```python
from build123d import *

# Parameters (mm, degrees)
FILLET1_R = 1.5


with BuildPart() as part:
    # Sketch1 → Revolve1 (revolve)
    with BuildSketch(Plane.XY):
        Polygon((33.75, 0), (33.75, -9), (13.25, -9), (13.25, -19), (0, -19), (0, -17), (11.25, -17), (11.25, -7), (31.75, -7), (31.75, 3), (32.75, 3), (32.75, 0), align=None)
    revolve(axis=Axis((0, -19, 0), (0, 1, 0)))

    # Fillet1
    fillet1_edges = [part.edges().sort_by_distance(p)[0] for p in [
        (-13.25, -19, 0),
        (-33.75, -9, 0),
    ]]
    fillet(fillet1_edges, radius=FILLET1_R)


solid = part.part
```
The listing builds one solid part. Answer for the finished solid, in the listing's coordinates (mm). A direction names the side the tool comes from. Coordinates: 2 decimals unless noted, no trailing zeros. Loops run counter-clockwise (first coordinate to the right, second up) from the corner with the lowest first, then second, coordinate; pieces in that order, holes last. Notation, with made-up numbers: (48, 8) -> (92, 8) arc R27 cw to (92, 27) -> close; hole circle Ø4 at (18.5, 13.5). An arc over 180 degrees is marked (long way). Use one line per item in the form item = value. Start each with the question number.
Item 1: A tool of negligible diameter and unlimited length cuts with its end or side. For faces 1 (the face through (0, -19, 0)), 2 (the face through (28, 0, -18)), 3 (the face through (14, -9, 0)), from which of +Z, -Z, +X, -X, +Y, -Y can it reach the whole face along a straight path? Write none if from no direction.
Item 2: The part is cut by section A-A on z = 0. Determine the outline of the cut face in (x, y).
Item 3: The part is cut by section C-C on y = -5.75. Determine the outline of the cut face in (x, z).
Item 4: The part is cut by section D-D on y = -11. Determine the outline of the cut face in (x, z).
Item 5: The mould has two halves that part along Z. Classify faces 4 (the face through (7.123, -13.31, -11.172)), 5 (the face through (0, -17, 0)), 6 (the face through (17, 3, -27)): released by +Z, released by -Z, zero draft, split by the parting line, or undercut.
Item 6: The part is cut by section B-B on x = 0. Determine the outline of the cut face in (y, z), then the cut area to 3 significant figures.
Item 7: Flat-ended cylindrical pins translate along their axes: pin 1 Ø6 at (y, z) = (0.5, 16) entering from -X; pin 2 Ø18 at (x, z) = (0, 0) entering from +Y; pin 3 Ø6 at (x, y) = (14.5, -10) entering from +Z. Find the tip coordinate at first contact, or state that the pin passes through.
Item 8: Consider L1, parallel to X at y = -13.5, z = 0; L2, parallel to Z at x = 0, y = -4. Determine where each line is inside the solid, lowest interval first. Write a range as [from, to].
Answer key:
q1.face_1 = +Z, -Z, +X, -X, -Y
q1.face_2 = +Y
q1.face_3 = -Y
q2.outline = (-33.75, -7.5) arc R1.5 ccw to (-32.25, -9) -> (-13.25, -9) -> (-13.25, -17.5) arc R1.5 ccw to (-11.75, -19) -> (11.75, -19) arc R1.5 ccw to (13.25, -17.5) -> (13.25, -9) -> (32.25, -9) arc R1.5 ccw to (33.75, -7.5) -> (33.75, 0) -> (32.75, 0) -> (32.75, 3) -> (31.75, 3) -> (31.75, -7) -> (11.25, -7) -> (11.25, -17) -> (-11.25, -17) -> (-11.25, -7) -> (-31.75, -7) -> (-31.75, 3) -> (-32.75, 3) -> (-32.75, 0) -> (-33.75, 0) -> close
q3.outline = circle Ø67.5 at (0, 0); hole circle Ø63.5 at (0, 0)
q4.outline = circle Ø26.5 at (0, 0); hole circle Ø22.5 at (0, 0)
q5.face_4 = split by the parting line
q5.face_5 = undercut
q5.face_6 = zero draft
q6.outline = (-19, -11.75) arc R1.5 ccw to (-17.5, -13.25) -> (-9, -13.25) -> (-9, -32.25) arc R1.5 ccw to (-7.5, -33.75) -> (0, -33.75) -> (0, -32.75) -> (3, -32.75) -> (3, -31.75) -> (-7, -31.75) -> (-7, -11.25) -> (-17, -11.25) -> (-17, 11.25) -> (-7, 11.25) -> (-7, 31.75) -> (3, 31.75) -> (3, 32.75) -> (0, 32.75) -> (0, 33.75) -> (-7.5, 33.75) arc R1.5 ccw to (-9, 32.25) -> (-9, 13.25) -> (-17.5, 13.25) arc R1.5 ccw to (-19, 11.75) -> close
q6.area = 207 mm2
q7.pin_1 = -31.13
q7.pin_2 = -17
q7.pin_3 = 31.35
q8.L1 = [-13.25, -11.25], [11.25, 13.25]
q8.L2 = [-33.75, -31.75], [31.75, 33.75]
